Geometry check sheet. Reference: the model listing, model coordinates, mm. Face numbers are marked on the shaded views. A direction names the side the tool comes from. Give positions to 0.01 mm unless a question says otherwise; leave off trailing zeros. Loops run counter-clockwise (first coordinate to the right, second up) from the corner with the lowest first, then second, coordinate; pieces in that order, holes last. Notation, with made-up numbers: (54.25, 1) - (88.25, 1) arc R20 ccw to (88.25, 36) - close; hole circle Ø9 at (21, 57). An arc over 180 degrees is marked (long way). Use a Markdown table: item, result. Add a question column.
1. Set-up check for the marked faces 1, 2, 3 and 4: record each of +Z, -Z, +X, -X, +Y, -Y from which the full face is reachable in a straight line by a thin tool's end or side.
2. Depth check by flat-ended pin: P1, Ø1.6, axis at x = 2, y = 52.5, coming from the -Z side; P2, Ø1, axis at x = 1.5, z = -16, coming from the -Y side; P3, Ø1.6, axis at x = 2, y = 7.5, coming from the +Z side. Enter the tip coordinate at first touch or a pass-through.
3. Cross-section at B-B on z = -5.5. Enter the section's corners in (x, y).
4. Cross-section at C-C on x = 1.5. Count the separate pieces of the cut face and the enclosed holes in it, and give its area (3 significant figures).
5. Cross-section at D-D on y = 52. Enter the section's corners in (x, z), and give its area (3 significant figures).
6. Draft check along Z on the marked faces 5, 6 and 7. Enter one of: pulls with the +Z half, pulls with the -Z half, needs draft (parallel to the pull), parting line crosses it, or undercut.
7. Cross-section at A-A on y = 24.7. Enter the section's corners in (x, z).
8. Material ranges on L1, parallel to Z at x = 1.5, y = 15.5; L2, parallel to Z at x = 1.2, y = 54.31; L3, parallel to Y at x = 0.9, z = -18.5, recorded low to high.
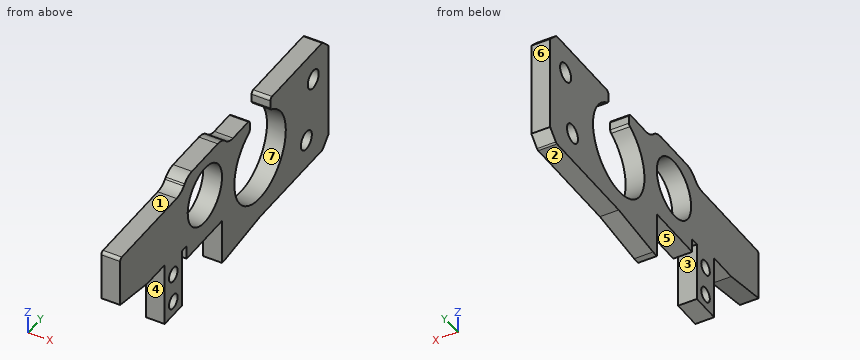
from build123d import *

# Parameters (mm, degrees)
SKETCH1_R           = 5
SKETCH1_R_2         = 1.6
SKETCH1_R_3         = 1.25
BOSS_EXTRUDE1_DEPTH = 3.18
CHAMFER1_SIZE       = 8
CHAMFER1_SIZE2      = 1.410615846
CUT_EXTRUDE5_DEPTH  = 65.412487143
FILLET2_R           = 3
CHAMFER3_SIZE       = 1
CHAMFER3_SIZE_2     = 10
CHAMFER2_SIZE       = 1.8
FILLET4_R           = 0.5


with BuildPart() as part:
    # Sketch1 → Boss-Extrude1 (new body)
    with BuildSketch(Plane(origin=(0, 0, 0), x_dir=(0, 0, -1), z_dir=(1, 0, 0))):
        Polygon((0, 0), (0, 17.7), (-2, 19.7), (-2, 29.7), (0, 31.7), (0, 60.81), (20, 60.81), (20, 40.81), (21, 40.81), (21, 29.68), (13.2, 29.68), (13.2, 19.4), (10.85, 19.4), (10.85, 18), (21, 18), (21, 13), (10, 13), (10, 0), align=None)
        with Locations(Location((5, 24.7, 0), (0, 0, 180))):
            Circle(SKETCH1_R, mode=Mode.SUBTRACT)
        with Locations(Location((5, 56.31, 0), (0, 0, 180))):
            Circle(SKETCH1_R_2, mode=Mode.SUBTRACT)
        with Locations(Location((15, 54.31, 0), (0, 0, 180))):
            Circle(SKETCH1_R_2, mode=Mode.SUBTRACT)
        with Locations(Location((18.5, 15.5, 0), (0, 0, 180))):
            Circle(SKETCH1_R_3, mode=Mode.SUBTRACT)
        with Locations(Location((13.5, 15.5, 0), (0, 0, 180))):
            Circle(SKETCH1_R_3, mode=Mode.SUBTRACT)
    extrude(amount=BOSS_EXTRUDE1_DEPTH)

    # Chamfer1
    chamfer1_edges = [part.edges().sort_by_distance(p)[0] for p in [
        (1.59, 0, -10),
    ]]
    chamfer1_side = [part.faces().sort_by_distance(p)[0] for p in [
        (1.59, 6.5, -10),
    ]]
    chamfer(chamfer1_edges, length=CHAMFER1_SIZE, length2=CHAMFER1_SIZE2, reference=chamfer1_side[0])

    # Sketch8 → Cut-Extrude5 (cut, through all)
    with BuildSketch(Plane(origin=(3.18, 0, 0), x_dir=(0, 0, -1), z_dir=(1, 0, 0))):
        with BuildLine():
            Line((0, 43.810865899), (2.126136458, 43.810865899))
            ThreePointArc((2.126136458, 43.810865899), (16.5, 40.810865899), (2.126136458, 37.810865899))
            Line((2.126136458, 37.810865899), (0, 37.810865899))
            Line((0, 37.810865899), (0, 43.810865899))
        make_face()
    extrude(amount=-CUT_EXTRUDE5_DEPTH, mode=Mode.SUBTRACT)

    # Fillet2
    fillet2_edges = [part.edges().sort_by_distance(p)[0] for p in [
        (1.59, 17.7, 0),
        (1.59, 19.7, 2),
        (1.59, 29.7, 2),
        (1.59, 31.7, 0),
    ]]
    fillet(fillet2_edges, radius=FILLET2_R)

    # Chamfer3
    # the kernel refuses this chamfer: 10, 1 mm, written as the material it takes off along each edge
    with BuildSketch(Plane(origin=(-25.99522763, 40.81, -21), x_dir=(0, 0.3574851447578462, 0.9339188247794675), z_dir=(1, 0, 0))) as chamfer3_piece_1:
        Polygon((CHAMFER3_SIZE * 0.933918824779, CHAMFER3_SIZE * 0.357485144758), (-CHAMFER3_SIZE_2 * 0.357485144758, CHAMFER3_SIZE_2 * 0.933918824779), (0, 0), align=None)
    extrude(amount=55.170455259, mode=Mode.SUBTRACT)

    # Chamfer2
    chamfer2_edges = [part.edges().sort_by_distance(p)[0] for p in [
        (1.59, 60.81, 0),
        (1.59, 60.81, -20),
    ]]
    chamfer(chamfer2_edges, length=CHAMFER2_SIZE)

    # Fillet4
    fillet4_edges = [part.edges().sort_by_distance(p)[0] for p in [
        (1.59, 59.01, -20),
        (1.59, 59.01, 0),
        (1.59, 0, 0),
        (1.59, 37.810865899, 0),
        (1.59, 43.810865899, 0),
        (1.59, 43.810865899, -2.126136458),
        (1.59, 37.810865899, -2.126136458),
    ]]
    fillet(fillet4_edges, radius=FILLET4_R)


solid = part.part
Values found:
| question | item | result |
|---|---|---|
| 1 | face 1 | +Z, +X, -X, -Y |
| 1 | face 2 | -Z, +X, -X, +Y |
| 1 | face 3 | -Z, +X, -X |
| 1 | face 4 | -Z, +X, -X, -Y |
| 2 | P1 | stops at z = -20 |
| 2 | P2 | stops at y = 13 |
| 2 | P3 | stops at z = 0 |
| 3 | outline | (0, 0) - (3.18, 0) - (3.18, 19.73) - (0, 19.73) - close; (0, 29.67) - (3.18, 29.67) - (3.18, 34.18) - (0, 34.18) - close; (0, 47.44) - (3.18, 47.44) - (3.18, 54.79) - (0, 54.79) - close; (0, 57.83) - (3.18, 57.83) - (3.18, 60.81) - (0, 60.81) - close |
| 4 | separate pieces | 1 |
| 4 | enclosed holes | 5 |
| 4 | area | 738 mm2 |
| 5 | outline | (0, -20) - (3.18, -20) - (3.18, 0) - (0, 0) - close |
| 5 | area | 63.6 mm2 |
| 6 | face 5 | pulls with the -Z half |
| 6 | face 6 | needs draft |
| 6 | face 7 | undercut |
| 7 | outline | (0, -13.2) - (3.18, -13.2) - (3.18, -10) - (0, -10) - close; (0, 0) - (3.18, 0) - (3.18, 2) - (0, 2) - close |
| 8 | L1 | z = -21 to -19.75, -17.25 to -14.75, -12.25 to 0 |
| 8 | L2 | z = -20 to -16.6, -13.4 to 0 |
| 8 | L3 | y = 13 to 14.25, 16.75 to 18, 29.68 to 60.51 |
